from build123d import *

# Parameters (mm, degrees)
SKETCH1_W           = 368.3
SKETCH1_H           = 50.8
BOSS_EXTRUDE1_DEPTH = 28.575
CHAMFER1_SIZE       = 6.35
FILLET1_R           = 3.175
SKETCH2_R           = 33.3375
CUT_EXTRUDE1_DEPTH  = 22.225
CUT_EXTRUDE2_REACH  = 190.186
CUT_EXTRUDE3_REACH  = 190.186
SKETCH5_W           = 6.604
SKETCH5_H           = 6.604
FILLET2_R           = 1.5875
CAVITY1_START       = 6.35
CAVITY1_OUTLINE_R   = 1.905
CAVITY1_DEPTH       = 22.225
CAVITY1_2_DEPTH     = 6.35
CUT_EXTRUDE4_REACH  = 188.943
SKETCH7_R           = 2.159


# Read off the part's stored shape, not the designer's step: Cavity1
with BuildPart() as part:
    # Sketch1 → Boss-Extrude1 (new body)
    with BuildSketch(Plane(origin=(0, 0, 0), x_dir=(0, 0, -1), z_dir=(1, 0, 0))):
        with Locations((0, 0.79375)):
            Rectangle(SKETCH1_W, SKETCH1_H)
    extrude(amount=BOSS_EXTRUDE1_DEPTH)

    # Chamfer1
    chamfer1_edges = [part.edges().sort_by_distance(p)[0] for p in [
        (14.2875, -24.60625, 184.15),
        (14.2875, -24.60625, -184.15),
    ]]
    chamfer(chamfer1_edges, length=CHAMFER1_SIZE)

    # Fillet1
    fillet1_edges = [part.edges().sort_by_distance(p)[0] for p in [
        (14.2875, -18.25625, -184.15),
        (14.2875, -24.60625, 177.8),
        (14.2875, -24.60625, -177.8),
        (14.2875, -18.25625, 184.15),
        (14.2875, 26.19375, 184.15),
        (14.2875, 26.19375, -184.15),
    ]]
    fillet(fillet1_edges, radius=FILLET1_R)

    # Sketch2 → Cut-Extrude1 (cut)
    with BuildSketch(Plane(origin=(28.575, 0, 0), x_dir=(0, 0, -1), z_dir=(1, 0, 0))):
        with Locations((-148.157911006, 0.79375)):
            Circle(SKETCH2_R)
        Circle(SKETCH2_R)
        with Locations((148.157911006, 0.79375)):
            Circle(SKETCH2_R)
    extrude(amount=-CUT_EXTRUDE1_DEPTH, mode=Mode.SUBTRACT)

    # Sketch4 → Cut-Extrude2 (cut, up to next)
    with BuildSketch(Plane(origin=(28.575, 0, 0), x_dir=(0, 0, -1), z_dir=(1, 0, 0)), mode=Mode.PRIVATE) as cut_extrude2_sk1:
        with BuildLine():
            ThreePointArc((-131.07672228, 10.893621573), (-168.001661006, 0.79375), (-131.07672228, -9.306121573))
            ThreePointArc((-131.07672228, -9.306121573), (-112.015493633, -20.636909552), (-93.124577673, -9.024395271))
            ThreePointArc((-93.124577673, -9.024395271), (-74.074577673, -20.6375), (-55.024577673, -9.024395271))
            ThreePointArc((-55.024577673, -9.024395271), (-36.370033983, -20.633851146), (-17.299823722, -9.720623089))
            ThreePointArc((-17.299823722, -9.720623089), (0, -19.84375), (17.299823722, -9.720623089))
            ThreePointArc((17.299823722, -9.720623089), (36.370033983, -20.633851146), (55.024577673, -9.024395271))
            ThreePointArc((55.024577673, -9.024395271), (74.074577673, -20.6375), (93.124577673, -9.024395271))
            ThreePointArc((93.124577673, -9.024395271), (112.015493633, -20.636909552), (131.07672228, -9.306121573))
            ThreePointArc((131.07672228, -9.306121573), (168.001661006, 0.79375), (131.07672228, 10.893621573))
            ThreePointArc((131.07672228, 10.893621573), (112.015493633, 22.224409552), (93.124577673, 10.611895271))
            ThreePointArc((93.124577673, 10.611895271), (74.074577673, 22.225), (55.024577673, 10.611895271))
            ThreePointArc((55.024577673, 10.611895271), (35.897270086, 22.224860566), (16.854241153, 10.474204945))
            ThreePointArc((16.854241153, 10.474204945), (0, 19.84375), (-16.854241153, 10.474204945))
            ThreePointArc((-16.854241153, 10.474204945), (-35.897270086, 22.224860566), (-55.024577673, 10.611895271))
            ThreePointArc((-55.024577673, 10.611895271), (-74.074577673, 22.225), (-93.124577673, 10.611895271))
            ThreePointArc((-93.124577673, 10.611895271), (-112.015493633, 22.224409552), (-131.07672228, 10.893621573))
        make_face()
    cut_extrude2_tool1 = extrude(cut_extrude2_sk1.sketch, amount=-CUT_EXTRUDE2_REACH, mode=Mode.PRIVATE) & part.part
    add(cut_extrude2_tool1.solids().sort_by_distance((28.575, 0.715797, 0))[0], mode=Mode.SUBTRACT)

    # Sketch5 → Cut-Extrude3 (cut, up to next)
    with BuildSketch(Plane(origin=(28.575, 0, 0), x_dir=(0, 0, -1), z_dir=(1, 0, 0)), mode=Mode.PRIVATE) as cut_extrude3_sk1:
        with Locations((-93.124577673, -18.322281394)):
            Rectangle(SKETCH5_W, SKETCH5_H)
    cut_extrude3_tool1 = extrude(cut_extrude3_sk1.sketch, amount=-CUT_EXTRUDE3_REACH, mode=Mode.PRIVATE) & part.part
    add(cut_extrude3_tool1.solids().sort_by_distance((28.575, -18.322281, 93.124578))[0], mode=Mode.SUBTRACT)

    # Fillet2
    fillet2_edges = [part.edges().sort_by_distance(p)[0] for p in [
        (17.4625, -24.60625, -169.750245438),
        (17.4625, 26.19375, -169.750245438),
        (17.4625, -24.60625, 169.750245438),
        (17.4625, 26.19375, 169.750245438),
    ]]
    fillet(fillet2_edges, radius=FILLET2_R)

    # Cavity1 outline → Cavity1 (cut)
    # profile 1 of 2: a face of its own
    with BuildSketch(Plane.YZ.offset(CAVITY1_START)):
        with BuildLine():
            ThreePointArc((-21.936363636, 172.545014982), (-20.786227921, 173.568410001), (-19.590070715, 174.537614554))
            ThreePointArc((-19.590070715, 174.537614554), (-16.522960019, 176.64510919), (-13.240070715, 178.397632936))
            ThreePointArc((-13.240070715, 178.397632936), (2.926403377, 181.427126443), (18.57375, 176.358274589))
            ThreePointArc((18.57375, 176.358274589), (21.138345447, 174.567877729), (23.523863636, 172.545014982))
            ThreePointArc((23.523863636, 172.545014982), (24.176019306, 172.178216056), (24.92375, 172.150879661))
            ThreePointArc((24.92375, 172.150879661), (25.835922212, 172.70228249), (26.19375, 173.706305647))
            Line((26.19375, 173.706305647), (26.19375, 180.975))
            ThreePointArc((26.19375, 180.975), (25.26381403, 183.22006403), (23.01875, 184.15))
            Line((23.01875, 184.15), (-16.941121939, 184.15))
            ThreePointArc((-16.941121939, 184.15), (-18.156141837, 183.908317516), (-19.18618597, 183.22006403))
            Line((-19.18618597, 183.22006403), (-23.67631403, 178.72993597))
            ThreePointArc((-23.67631403, 178.72993597), (-24.364567516, 177.699891837), (-24.60625, 176.484871939))
            Line((-24.60625, 176.484871939), (-24.60625, 173.706305647))
            ThreePointArc((-24.60625, 173.706305647), (-23.651943453, 172.250550757), (-21.936363636, 172.545014982))
        make_face()
        with Locations((-16.415070715, 179.705)):
            Circle(CAVITY1_OUTLINE_R, mode=Mode.SUBTRACT)
        with Locations((21.74875, 179.705)):
            Circle(CAVITY1_OUTLINE_R, mode=Mode.SUBTRACT)
    # profile 2 of 2: a face of its own
    with BuildSketch(Plane.YZ.offset(CAVITY1_START)):
        with BuildLine():
            ThreePointArc((-21.936363636, -172.545014982), (-23.651943453, -172.250550757), (-24.60625, -173.706305647))
            Line((-24.60625, -173.706305647), (-24.60625, -176.484871939))
            ThreePointArc((-24.60625, -176.484871939), (-24.364567516, -177.699891837), (-23.67631403, -178.72993597))
            Line((-23.67631403, -178.72993597), (-19.18618597, -183.22006403))
            ThreePointArc((-19.18618597, -183.22006403), (-18.156141837, -183.908317516), (-16.941121939, -184.15))
            Line((-16.941121939, -184.15), (23.01875, -184.15))
            ThreePointArc((23.01875, -184.15), (25.26381403, -183.22006403), (26.19375, -180.975))
            Line((26.19375, -180.975), (26.19375, -173.706305647))
            ThreePointArc((26.19375, -173.706305647), (25.835922212, -172.70228249), (24.92375, -172.150879661))
            ThreePointArc((24.92375, -172.150879661), (24.176019306, -172.178216056), (23.523863636, -172.545014982))
            ThreePointArc((23.523863636, -172.545014982), (21.138345447, -174.567877729), (18.57375, -176.358274589))
            ThreePointArc((18.57375, -176.358274589), (2.926403377, -181.427126443), (-13.240070715, -178.397632935))
            ThreePointArc((-13.240070715, -178.397632935), (-16.522960019, -176.64510919), (-19.590070715, -174.537614554))
            ThreePointArc((-19.590070715, -174.537614554), (-20.786227921, -173.568410001), (-21.936363636, -172.545014982))
        make_face()
        with Locations((-16.415070715, -179.705)):
            Circle(CAVITY1_OUTLINE_R, mode=Mode.SUBTRACT)
        with Locations((21.74875, -179.705)):
            Circle(CAVITY1_OUTLINE_R, mode=Mode.SUBTRACT)
    extrude(amount=CAVITY1_DEPTH, mode=Mode.SUBTRACT)

    # Cavity1 2 outline → Cavity1 2 (cut)
    with BuildSketch(Plane.YZ):
        with BuildLine():
            Line((-13.240070715, 179.705), (-13.240070715, 178.397632935))
            ThreePointArc((-13.240070715, 178.397632935), (2.926403377, 181.427126443), (18.57375, 176.358274589))
            Line((18.57375, 176.358274589), (18.57375, 179.705))
            ThreePointArc((18.57375, 179.705), (21.74875, 182.88), (24.92375, 179.705))
            Line((24.92375, 179.705), (24.92375, 172.150879661))
            ThreePointArc((24.92375, 172.150879661), (25.835922212, 172.70228249), (26.19375, 173.706305647))
            Line((26.19375, 173.706305647), (26.19375, 180.975))
            ThreePointArc((26.19375, 180.975), (25.26381403, 183.22006403), (23.01875, 184.15))
            Line((23.01875, 184.15), (-16.941121939, 184.15))
            ThreePointArc((-16.941121939, 184.15), (-18.156141837, 183.908317516), (-19.18618597, 183.22006403))
            Line((-19.18618597, 183.22006403), (-23.67631403, 178.72993597))
            ThreePointArc((-23.67631403, 178.72993597), (-24.364567516, 177.699891837), (-24.60625, 176.484871939))
            Line((-24.60625, 176.484871939), (-24.60625, 173.706305647))
            ThreePointArc((-24.60625, 173.706305647), (-23.651943453, 172.250550757), (-21.936363636, 172.545014982))
            ThreePointArc((-21.936363636, 172.545014982), (-20.786227921, 173.568410001), (-19.590070715, 174.537614554))
            Line((-19.590070715, 174.537614554), (-19.590070715, 179.705))
            ThreePointArc((-19.590070715, 179.705), (-16.415070715, 182.88), (-13.240070715, 179.705))
        make_face()
        with BuildLine():
            ThreePointArc((-21.936363636, -172.545014982), (-23.651943453, -172.250550757), (-24.60625, -173.706305647))
            Line((-24.60625, -173.706305647), (-24.60625, -176.484871939))
            ThreePointArc((-24.60625, -176.484871939), (-24.364567516, -177.699891837), (-23.67631403, -178.72993597))
            Line((-23.67631403, -178.72993597), (-19.18618597, -183.22006403))
            ThreePointArc((-19.18618597, -183.22006403), (-18.156141837, -183.908317516), (-16.941121939, -184.15))
            Line((-16.941121939, -184.15), (23.01875, -184.15))
            ThreePointArc((23.01875, -184.15), (25.26381403, -183.22006403), (26.19375, -180.975))
            Line((26.19375, -180.975), (26.19375, -173.706305647))
            ThreePointArc((26.19375, -173.706305647), (25.835922212, -172.70228249), (24.92375, -172.150879661))
            Line((24.92375, -172.150879661), (24.92375, -179.705))
            ThreePointArc((24.92375, -179.705), (21.74875, -182.88), (18.57375, -179.705))
            Line((18.57375, -179.705), (18.57375, -176.358274589))
            ThreePointArc((18.57375, -176.358274589), (2.926403377, -181.427126443), (-13.240070715, -178.397632935))
            Line((-13.240070715, -178.397632935), (-13.240070715, -179.705))
            ThreePointArc((-13.240070715, -179.705), (-16.415070715, -182.88), (-19.590070715, -179.705))
            Line((-19.590070715, -179.705), (-19.590070715, -174.537614554))
            ThreePointArc((-19.590070715, -174.537614554), (-20.786227921, -173.568410001), (-21.936363636, -172.545014982))
        make_face()
    extrude(amount=CAVITY1_2_DEPTH, mode=Mode.SUBTRACT)

    # Sketch7 → Cut-Extrude4 (cut, up to next)
    with BuildSketch(Plane(origin=(28.575, 0, 0), x_dir=(0, 0, -1), z_dir=(1, 0, 0)), mode=Mode.PRIVATE) as cut_extrude4_sk1:
        with Locations((-179.705, 21.74875)):
            Circle(SKETCH7_R)
    cut_extrude4_tool1 = extrude(cut_extrude4_sk1.sketch, amount=-CUT_EXTRUDE4_REACH, mode=Mode.PRIVATE) & part.part
    # Sketch7 → Cut-Extrude4 (cut, up to next)
    with BuildSketch(Plane(origin=(28.575, 0, 0), x_dir=(0, 0, -1), z_dir=(1, 0, 0)), mode=Mode.PRIVATE) as cut_extrude4_sk2:
        with Locations((-179.705, -16.415070715)):
            Circle(SKETCH7_R)
    cut_extrude4_tool2 = extrude(cut_extrude4_sk2.sketch, amount=-CUT_EXTRUDE4_REACH, mode=Mode.PRIVATE) & part.part
    # Sketch7 → Cut-Extrude4 (cut, up to next)
    with BuildSketch(Plane(origin=(28.575, 0, 0), x_dir=(0, 0, -1), z_dir=(1, 0, 0)), mode=Mode.PRIVATE) as cut_extrude4_sk3:
        with Locations((179.705, 21.74875)):
            Circle(SKETCH7_R)
    cut_extrude4_tool3 = extrude(cut_extrude4_sk3.sketch, amount=-CUT_EXTRUDE4_REACH, mode=Mode.PRIVATE) & part.part
    # Sketch7 → Cut-Extrude4 (cut, up to next)
    with BuildSketch(Plane(origin=(28.575, 0, 0), x_dir=(0, 0, -1), z_dir=(1, 0, 0)), mode=Mode.PRIVATE) as cut_extrude4_sk4:
        with Locations((179.705, -16.415070715)):
            Circle(SKETCH7_R)
    cut_extrude4_tool4 = extrude(cut_extrude4_sk4.sketch, amount=-CUT_EXTRUDE4_REACH, mode=Mode.PRIVATE) & part.part
    add(cut_extrude4_tool1.solids().sort_by_distance((28.575, 21.74875, 179.705))[0], mode=Mode.SUBTRACT)
    add(cut_extrude4_tool2.solids().sort_by_distance((28.575, -16.415071, 179.705))[0], mode=Mode.SUBTRACT)
    add(cut_extrude4_tool3.solids().sort_by_distance((28.575, 21.74875, -179.705))[0], mode=Mode.SUBTRACT)
    add(cut_extrude4_tool4.solids().sort_by_distance((28.575, -16.415071, -179.705))[0], mode=Mode.SUBTRACT)


solid = part.part
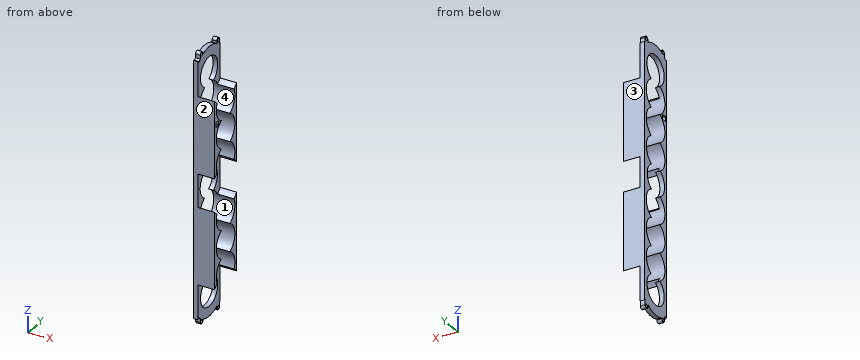
Geometry check sheet. Reference: the model listing, model coordinates, mm. Face numbers are marked on the shaded views. A direction names the side the tool comes from. Coordinates: 2 decimals unless noted, no trailing zeros. Write each loop counter-clockwise with the first axis right and the second up, starting at its lowest first coordinate (ties: lowest second). Pieces come first, ordered by that corner, then holes. Notation, with made-up numbers: (-13, 31) -> (22, 31) arc R22 ccw to (22, 39) -> close; hole circle Ø8 at (49, 8.5). An arc over 180 degrees is marked (long way). One line per question, with ' | ' between items.
1. Cross-section at B-B on z = 67.5. Record the cut outline in (x, y) (3 decimals).
Answers:
outline: (0, -24.606) -> (28.575, -24.606) -> (28.575, -19.604) -> (0, -19.604) -> close; (0, 21.192) -> (28.575, 21.192) -> (28.575, 26.194) -> (0, 26.194) -> close
2. Cross-section at A-A on x = 21.75. Record the cut outline in (y, z) (1 decimal), and give its area (3 significant figures).
Answers:
outline: (-24.6, -126.6) arc R33.3 cw to (-18.7, -121.1) arc R21.4 cw to (-9, -93.1) arc R21.4 cw to (-9, -55) arc R21.4 cw to (-18.9, -27.5) arc R33.3 cw to (-24.6, -22.5) -> close; (-24.6, 22.5) arc R33.3 cw to (-18.9, 27.5) arc R21.4 cw to (-9, 55) arc R21.4 cw to (-9, 93.1) arc R21.4 cw to (-18.7, 121.1) arc R33.3 cw to (-24.6, 126.6) -> close; (10.6, -93.1) arc R21.4 cw to (20.3, -121.1) arc R33.3 cw to (26.2, -126.6) -> (26.2, -20.6) arc R33.3 cw to (20.1, -26.6) arc R21.4 cw to (10.6, -55) arc R21.4 cw to start; (10.6, 55) arc R21.4 cw to (20.1, 26.6) arc R33.3 cw to (26.2, 20.6) -> (26.2, 126.6) arc R33.3 cw to (20.3, 121.1) arc R21.4 cw to (10.6, 93.1) arc R21.4 cw to start; hole (-21.6, 89.8) -> (-15, 89.8) -> (-15, 96.4) -> (-21.6, 96.4) -> close | area: 2,630 mm²
3. Depth check by flat-ended pin: pin 1 Ø5 at (x, z) = (4, -177.5) entering from +Y; pin 2 Ø10 at (x, y) = (12.5, 4) entering from -Z; pin 3 Ø8 at (y, z) = (17.5, -13) entering from +X; pin 4 Ø2.5 at (x, z) = (2.5, -177.5) entering from -Y. Enter the tip coordinate at first touch or a pass-through.
Answers:
pin 1: stops at y = 24.92 | pin 2: passes through | pin 3: stops at x = 6.35 | pin 4: stops at y = -19.59
4. Thickness scan on probe 1 along Z at (x, y) = (8.75, -17.5); probe 2 along Z at (x, y) = (21, 13); probe 3 along Z at (x, y) = (19.5, 15). Record the ranges inside material, lowest first. Write a range as from..to.
Answers:
probe 1: z = -101.01..-85.24, -62.91..-47.14, 47.14..62.91, 85.24..89.82, 96.43..101.01 | probe 2: z = -94.56..-91.69, -56.46..-53.59, 53.59..56.46, 91.69..94.56 | probe 3: z = -96.13..-90.12, -58.03..-52.02, 52.02..58.03, 90.12..96.13
5. Cross-section at C-C on y = -4. Record the cut outline in (x, z).
Answers:
outline: (0, -181.15) -> (6.35, -181.15) -> (6.35, -167.41) -> (0, -167.41) -> close; (0, 167.41) -> (6.35, 167.41) -> (6.35, 181.15) -> (0, 181.15) -> close
6. Draft check along Z on the marked faces 1 and 2. Enter one of: +Z half, -Z half, draft (parallel to the pull), parting line (faces both ways), or undercut.
Answers:
face 1: undercut | face 2: draft
7. Set-up check for the marked faces 3 and 4: record each of +Z, -Z, +X, -X, +Y, -Y from which the full face is reachable in a straight line by a thin tool's end or side.
Answers:
face 3: +Z, -Z, +X, -X, +Y | face 4: +X, -X
